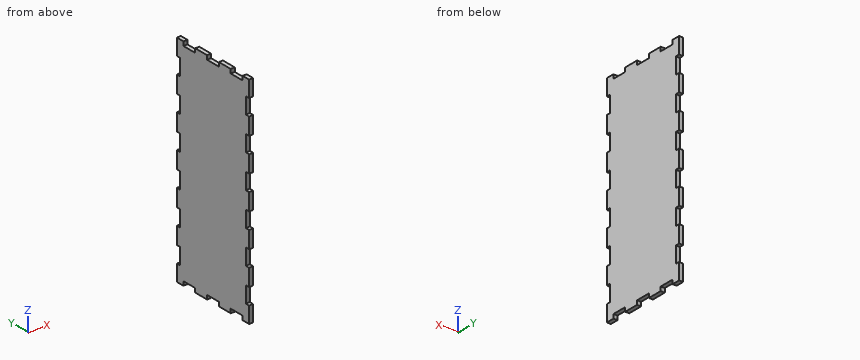
```python
from build123d import *

# Parameters (mm, degrees)
SKETCH1_W           = 265
SKETCH1_H           = 110
BOSS_EXTRUDE1_DEPTH = 5
SKETCH2_W           = 5
SKETCH2_H           = 18
SKETCH2_W_2         = 20
SKETCH2_H_2         = 5
CUT_EXTRUDE1_DEPTH  = 5


with BuildPart() as part:
    # Sketch1 → Boss-Extrude1 (new body)
    with BuildSketch(Plane(origin=(0, 0, 0), x_dir=(0, 0, -1), z_dir=(1, 0, 0))):
        Rectangle(SKETCH1_W, SKETCH1_H)
    extrude(amount=BOSS_EXTRUDE1_DEPTH)

    # Sketch2 → Cut-Extrude1 (cut)
    with BuildSketch(Plane(origin=(5, 0, 0), x_dir=(0, 0, -1), z_dir=(1, 0, 0))):
        with Locations((-130, 36)):
            Rectangle(SKETCH2_W, SKETCH2_H)
        with Locations((-130, 0)):
            Rectangle(SKETCH2_W, SKETCH2_H)
        with Locations((-130, -36)):
            Rectangle(SKETCH2_W, SKETCH2_H)
        with Locations((130, -36)):
            Rectangle(SKETCH2_W, SKETCH2_H)
        with Locations((130, 0)):
            Rectangle(SKETCH2_W, SKETCH2_H)
        with Locations((130, 36)):
            Rectangle(SKETCH2_W, SKETCH2_H)
        with Locations((-61.5, 52.5)):
            Rectangle(SKETCH2_W_2, SKETCH2_H_2)
        with Locations((-102.5, 52.5)):
            Rectangle(SKETCH2_W_2, SKETCH2_H_2)
        with Locations((-20.5, 52.5)):
            Rectangle(SKETCH2_W_2, SKETCH2_H_2)
        with Locations((20.5, 52.5)):
            Rectangle(SKETCH2_W_2, SKETCH2_H_2)
        with Locations((61.5, 52.5)):
            Rectangle(SKETCH2_W_2, SKETCH2_H_2)
        with Locations((102.5, 52.5)):
            Rectangle(SKETCH2_W_2, SKETCH2_H_2)
        with Locations((102.5, -52.5)):
            Rectangle(SKETCH2_W_2, SKETCH2_H_2)
        with Locations((61.5, -52.5)):
            Rectangle(SKETCH2_W_2, SKETCH2_H_2)
        with Locations((20.5, -52.5)):
            Rectangle(SKETCH2_W_2, SKETCH2_H_2)
        with Locations((-20.5, -52.5)):
            Rectangle(SKETCH2_W_2, SKETCH2_H_2)
        with Locations((-61.5, -52.5)):
            Rectangle(SKETCH2_W_2, SKETCH2_H_2)
        with Locations((-102.5, -52.5)):
            Rectangle(SKETCH2_W_2, SKETCH2_H_2)
    extrude(amount=-CUT_EXTRUDE1_DEPTH, mode=Mode.SUBTRACT)


solid = part.part
```
Check sheet for the modelled part. Datum: model origin and axes. Units: mm. Coordinates: 2 decimals unless noted, no trailing zeros. Order: outer loops, then holes, each group sorted by start corner. A loop starts at its lowest first (then second) coordinate and runs counter-clockwise, first axis right, second up. Notation, with made-up numbers: (22, 34.25) -> (40, 34.25) arc R32 ccw to (40, 69.25) -> close; hole circle Ø5 at (-18.75, -11.5). An arc over 180 degrees is marked (long way). Write each question's results on one line, items separated by ' | '. Start each with the question number.
1) Depth check by flat-ended pin: pin 1 (1.5 mm diameter, centred on x = 3.5, y = 40.5, fed in from -Z); pin 2 (2.5 mm diameter, centred on x = 3.5, z = 65.5, fed in from +Y); pin 3 (2.5 mm diameter, centred on x = 3.5, z = -64.5, fed in from -Y). Enter the tip coordinate at first touch or a pass-through.
2) Section check A-A (y = -6.5). Enter the section's corners in (x, z).
3) Material ranges on line 1 along Y through (x, z) = (4.25, -64.5); line 2 along Z through (x, y) = (4.75, -28.5), recorded low to high.
4) Section check B-B (z = -98). Enter the section's corners in (x, y).
Checked values:
1) pin 1: z = -127.5 | pin 2: y = 50 | pin 3: y = -50
2) outline: (0, -127.5) -> (5, -127.5) -> (5, 127.5) -> (0, 127.5) -> close
3) line 1: -50 to 50 | line 2: -127.5 to 127.5
4) outline: (0, -50) -> (5, -50) -> (5, 50) -> (0, 50) -> close
